The listing builds one solid part. Answer for the finished solid, in the listing's coordinates (mm). Face numbers are marked on the shaded views. A direction names the side the tool comes from. Give positions to 0.01 mm unless a question says otherwise; leave off trailing zeros. Loops run counter-clockwise (first coordinate to the right, second up) from the corner with the lowest first, then second, coordinate; pieces in that order, holes last.
Item 1: Section D-D, the plane y = 18 is taken. Give the vertices of the cut face in (x, z), and give its area (3 significant figures).
Item 2: Each of these flat-tipped pins is pushed along its axis until it touches: pin 1 Ø5 at (y, z) = (19, 21.5) entering from +X; pin 2 Ø8 at (y, z) = (15, 9) entering from -X; pin 3 Ø6.5 at (x, y) = (0, -28.575) entering from -Z. Where does it stop, or does it pass through?
Item 3: A tool of negligible diameter and unlimited length cuts with its end or side. For the marked faces 1, 2 and 3, from which of +Z, -Z, +X, -X, +Y, -Y can it reach the whole face along a straight path? Write none if from no direction.
Item 4: Section A-A, the plane y = 0 is taken. Give the vertices of the cut face in (x, z), and give its area (3 significant figures).
Item 5: Consider line 1 along Y through (x, z) = (0, 4.6); line 2 along Y through (x, z) = (0, 22); line 3 along Y through (x, z) = (0.5, 15). Determine where each line is inside the solid, lowest interval first.
Item 6: The mould has two halves that part along X. Classify the marked faces 4, 5 and 6: pulls with the +X half, pulls with the -X half, needs draft (parallel to the pull), parting line crosses it, or undercut.
Item 7: Section C-C, the plane z = 16.25 is taken. Give the vertices of the cut face in (x, y), and give its area (3 significant figures).
Item 8: Section B-B, the plane y = -11.5 is taken. Give the vertices of the cut face in (x, z).
from build123d import *

# Parameters (mm, degrees)
SKETCH1_R                       = 31.75
BOSS_EXTRUDE1_DEPTH             = 25.4
SKETCH2_OUTSIDE_W               = 84.166
SKETCH2_OUTSIDE_H               = 84.166
SKETCH2_OUTSIDE_R               = 18.796
CUT_EXTRUDE1_DEPTH              = 19.05
SKETCH3_R                       = 12.7
CUT_EXTRUDE2_DEPTH              = 26.4
F_2_56_TAPPED_HOLE1_D           = 1.778
F_2_56_TAPPED_HOLE1_DEPTH       = 5.73278
F_2_56_TAPPED_HOLE1_TIP         = 0.53416509
F_5_32_0_15625_DIAMETER_HOLE1_D = 3.96875
MIRROR2_COPY_1_D                = 3.96875
MIRROR2_COPY_2_D                = 3.96875
CUT_EXTRUDE3_DEPTH              = 26.4
CIRPATTERN1_COUNT               = 3
SKETCH10_R                      = 10.16
SKETCH10_R_2                    = 7.9375
CUT_EXTRUDE4_DEPTH              = 3.175


with BuildPart() as part:
    # Sketch1 → Boss-Extrude1 (new body)
    with BuildSketch(Plane.XY):
        Circle(SKETCH1_R)
    extrude(amount=BOSS_EXTRUDE1_DEPTH)

    # Sketch2 outside → Cut-Extrude1 (cut)
    with BuildSketch(Plane(origin=(0, 0, 0), x_dir=(-1, 0, 0), z_dir=(0, 0, -1))):
        Rectangle(SKETCH2_OUTSIDE_W, SKETCH2_OUTSIDE_H)
        Circle(SKETCH2_OUTSIDE_R, mode=Mode.SUBTRACT)
    extrude(amount=-CUT_EXTRUDE1_DEPTH, mode=Mode.SUBTRACT)

    # Sketch3 → Cut-Extrude2 (cut, through all)
    with BuildSketch(Plane(origin=(0, 0, 0), x_dir=(-1, 0, 0), z_dir=(0, 0, -1))):
        Circle(SKETCH3_R)
    extrude(amount=-CUT_EXTRUDE2_DEPTH, mode=Mode.SUBTRACT)

    # #2-56 Tapped Hole1
    with Locations(Plane(origin=(0, 0, 0), x_dir=(-1, 0, 0), z_dir=(0, 0, -1))):
        with Locations((0, 15.24), (0, -15.24)):
            Hole(F_2_56_TAPPED_HOLE1_D / 2, depth=F_2_56_TAPPED_HOLE1_DEPTH)
            with Locations((0, 0, -(F_2_56_TAPPED_HOLE1_DEPTH + F_2_56_TAPPED_HOLE1_TIP / 2))):  # 118° drill point
                Cone(0, F_2_56_TAPPED_HOLE1_D / 2, F_2_56_TAPPED_HOLE1_TIP, mode=Mode.SUBTRACT)

    # 5/32 (0.15625) Diameter Hole1 (through all)
    with Locations(Plane.XY.offset(25.4)):
        with Locations((0, 28.575), (28.575, 0)):
            f_5_32_0_15625_diameter_hole1 = Hole(F_5_32_0_15625_DIAMETER_HOLE1_D / 2)

    # Mirror1: 5/32 (0.15625) Diameter Hole1 across plane
    add(f_5_32_0_15625_diameter_hole1.mirror(Plane.ZX), mode=Mode.SUBTRACT)

    # Mirror2 copy 1 (through all)
    with Locations(Plane(origin=(0, 0, 25.4), x_dir=(-1, 0, 0), z_dir=(0, 0, 1))):
        with Locations((0, 28.575), (28.575, 0)):
            Hole(MIRROR2_COPY_1_D / 2)

    # Mirror2 copy 2 (through all)
    with Locations(Plane(origin=(0, 0, 25.4), x_dir=(-1, 0, 0), z_dir=(0, 0, 1))):
        with Locations((0, -28.575), (28.575, 0)):
            Hole(MIRROR2_COPY_2_D / 2)

    # Sketch9 → Cut-Extrude3 (cut, through all)
    with BuildSketch(Plane.XY.offset(25.4)):
        with BuildLine():
            ThreePointArc((17.520714904, 16.278611836), (11.957933079, 20.711747646), (5.337333936, 23.312690118))
            ThreePointArc((5.337333936, 23.312690118), (2.551061387, 21.564550521), (4.299200984, 18.778277972))
            ThreePointArc((4.299200984, 18.778277972), (9.632066921, 16.683229289), (14.112865271, 13.112356254))
            ThreePointArc((14.112865271, 13.112356254), (17.399917879, 12.991559228), (17.520714904, 16.278611836))
        make_face()
    cut_extrude3 = extrude(amount=-CUT_EXTRUDE3_DEPTH, mode=Mode.SUBTRACT)

    # CirPattern1: Cut-Extrude3 ×3 about axis
    cirpattern1_axis = Axis((0, 0, 0), (0, 0, 1))
    for i in range(1, CIRPATTERN1_COUNT):
        add(cut_extrude3.rotate(cirpattern1_axis, i * 360 / CIRPATTERN1_COUNT), mode=Mode.SUBTRACT)

    # Sketch10 → Cut-Extrude4 (cut)
    with BuildSketch(Plane(origin=(0, 0, 0), x_dir=(-1, 0, 0), z_dir=(0, 0, -1))):
        Circle(SKETCH10_R)
        Circle(SKETCH10_R_2, mode=Mode.SUBTRACT)
    extrude(amount=-CUT_EXTRUDE4_DEPTH, mode=Mode.SUBTRACT)


solid = part.part
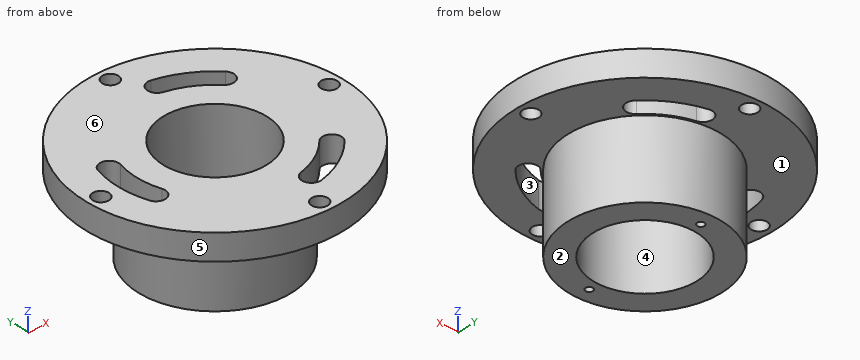
Worked answers:
1. outline: (-26.15, 19.05) - (-5.41, 19.05) - (-5.41, 0) - (5.41, 0) - (5.41, 19.05) - (6.86, 19.05) - (6.86, 25.4) - (-26.15, 25.4) - close; (15.75, 19.05) - (26.15, 19.05) - (26.15, 25.4) - (15.75, 25.4) - close
1. area: 482 mm2
2. pin 1: stops at x = 27.13
2. pin 2: stops at x = -15.24
2. pin 3: stops at z = 19.05
3. face 1: -Z
3. face 2: -Z, +X, -X, +Y, -Y
3. face 3: +Z, -Z
4. outline: (-31.75, 19.05) - (-30.56, 19.05) - (-30.56, 25.4) - (-31.75, 25.4) - close; (-26.59, 19.05) - (-23.92, 19.05) - (-23.92, 25.4) - (-26.59, 25.4) - close; (-19.26, 19.05) - (-18.8, 19.05) - (-18.8, 0) - (-12.7, 0) - (-12.7, 25.4) - (-19.26, 25.4) - close; (12.7, 0) - (18.8, 0) - (18.8, 19.05) - (26.59, 19.05) - (26.59, 25.4) - (12.7, 25.4) - close; (30.56, 19.05) - (31.75, 19.05) - (31.75, 25.4) - (30.56, 25.4) - close
4. area: 394 mm2
5. line 1: y = -18.8 to -16.13, -14.35 to -12.7, 12.7 to 14.35, 16.13 to 18.8
5. line 2: y = -31.75 to -30.56, -26.59 to -12.7, 12.7 to 26.59, 30.56 to 31.75
5. line 3: y = -18.79 to -12.69, 12.69 to 18.79
6. face 4: undercut
6. face 5: parting line crosses it
6. face 6: needs draft
7. outline: circle Ø37.59 at (0, 0); hole circle Ø25.4 at (0, 0)
7. area: 603 mm2
8. outline: (-29.59, 19.05) - (-14.87, 19.05) - (-14.87, 0) - (-5.39, 0) - (-5.39, 25.4) - (-29.59, 25.4) - close; (5.39, 0) - (14.87, 0) - (14.87, 19.05) - (29.59, 19.05) - (29.59, 25.4) - (5.39, 25.4) - close
